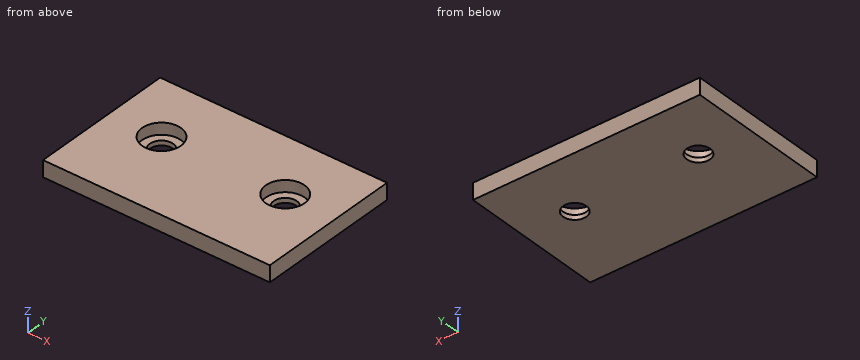
from build123d import *

# Parameters (mm, degrees)
CROQUIS1_W                                           = 69.85
CROQUIS1_H                                           = 44.45
SALIENTE_EXTRUIR1_DEPTH                              = 5
REFRENTADO_PARA_TORNILLO_CON_CABEZA_HUEC_D           = 7.14248
REFRENTADO_PARA_TORNILLO_CON_CABEZA_HUEC_DEPTH       = 24
REFRENTADO_PARA_TORNILLO_CON_CABEZA_HUEC_CBORE_D     = 11.938
REFRENTADO_PARA_TORNILLO_CON_CABEZA_HUEC_CBORE_DEPTH = 3.556
REFRENTADO_PARA_TORNILLO_CON_CABEZA_HUEC_TIP         = 2.145817477


with BuildPart() as part:
    # Croquis1 → Saliente-Extruir1 (new body)
    with BuildSketch(Plane.XY):
        Rectangle(CROQUIS1_W, CROQUIS1_H)
    extrude(amount=-SALIENTE_EXTRUIR1_DEPTH)

    # Refrentado para tornillo con cabeza hueca de 1/42
    with Locations(Plane.XY):
        with Locations((-19.05, 3.175), (19.05, 3.175)):
            CounterBoreHole(REFRENTADO_PARA_TORNILLO_CON_CABEZA_HUEC_D / 2, REFRENTADO_PARA_TORNILLO_CON_CABEZA_HUEC_CBORE_D / 2, REFRENTADO_PARA_TORNILLO_CON_CABEZA_HUEC_CBORE_DEPTH, depth=REFRENTADO_PARA_TORNILLO_CON_CABEZA_HUEC_DEPTH)
            with Locations((0, 0, -(REFRENTADO_PARA_TORNILLO_CON_CABEZA_HUEC_DEPTH + REFRENTADO_PARA_TORNILLO_CON_CABEZA_HUEC_TIP / 2))):  # 118° drill point
                Cone(0, REFRENTADO_PARA_TORNILLO_CON_CABEZA_HUEC_D / 2, REFRENTADO_PARA_TORNILLO_CON_CABEZA_HUEC_TIP, mode=Mode.SUBTRACT)


solid = part.part
Geometry: final body of the model. Coordinates: model frame, mm. Coordinates: 2 decimals unless noted, no trailing zeros. Write each loop counter-clockwise with the first axis right and the second up, starting at its lowest first coordinate (ties: lowest second). Pieces come first, ordered by that corner, then holes. Notation, with made-up numbers: (24, -33.5) - (81, -33.5) arc R16 cw to (81, -21.5) - close; hole circle Ø8 at (35.25, 65.25). An arc over 180 degrees is marked (long way). Return JSON: item names as keys, results as strings.
Item 1: Section query D-D (z = -2.8). Output: boundary loops of the cut face in (x, y) (3 decimals).
Completed:
{"outline": "(-34.925, -22.225) - (34.925, -22.225) - (34.925, 22.225) - (-34.925, 22.225) - close; hole circle Ø11.938 at (-19.05, 3.175); hole circle Ø11.938 at (19.05, 3.175)"}
Item 2: Section query B-B (y = 5). Output: boundary loops of the cut face in (x, z) (3 decimals).
Completed:
{"outline": "(-34.925, -5) - (-22.12, -5) - (-22.12, -3.556) - (-24.733, -3.556) - (-24.733, 0) - (-34.925, 0) - close; (-15.98, -5) - (15.98, -5) - (15.98, -3.556) - (13.367, -3.556) - (13.367, 0) - (-13.367, 0) - (-13.367, -3.556) - (-15.98, -3.556) - close; (22.12, -5) - (34.925, -5) - (34.925, 0) - (24.733, 0) - (24.733, -3.556) - (22.12, -3.556) - close"}
Item 3: Line query: L1, parallel to X at y = -0.5, z = -1.1 (3 decimals); L2, parallel to Y at x = -19.05, z = -4.5 (3 decimals); L3, parallel to Y at x = -19.05, z = -1.1 (3 decimals). Output: solid intervals per line, ascending.
Completed:
{"L1": "x = -34.925 to -23.754, -14.346 to 14.346, 23.754 to 34.925", "L2": "y = -22.225 to -0.396, 6.746 to 22.225", "L3": "y = -22.225 to -2.794, 9.144 to 22.225"}
Item 4: Pin query (flat end, axial travel): pin 1 Ø1.5 at (x, y) = (22.5, 6) entering from +Z. Return the tip coordinate at first contact, or that it passes through.
Completed:
{"pin 1": "stops at z = -3.56"}
Item 5: Section query C-C (x = -17). Output: boundary loops of the cut face in (y, z) (3 decimals).
Completed:
{"outline": "(-22.225, -5) - (0.251, -5) - (0.251, -3.556) - (-2.431, -3.556) - (-2.431, 0) - (-22.225, 0) - close; (6.099, -5) - (22.225, -5) - (22.225, 0) - (8.781, 0) - (8.781, -3.556) - (6.099, -3.556) - close"}
Item 6: Section query A-A (x = 19.05). Output: boundary loops of the cut face in (y, z) (3 decimals).
Completed:
{"outline": "(-22.225, -5) - (-0.396, -5) - (-0.396, -3.556) - (-2.794, -3.556) - (-2.794, 0) - (-22.225, 0) - close; (6.746, -5) - (22.225, -5) - (22.225, 0) - (9.144, 0) - (9.144, -3.556) - (6.746, -3.556) - close"}
